Autodesk Inventor part; units mm, degrees
ref_plane "Work Plane1" through (0, 0, -15) normal (0, 0, 1) x (1, 0, 0)
ref_plane "YZ Plane" through (0, 0, 0) normal (1, 0, 0) x (0, 1, 0)
ref_plane "XZ Plane" through (0, 0, 0) normal (0, 1, 0) x (-1, 0, 0)
sketch "Sketch1" plane through (0, 0, 0) normal (0, 0, 1) x (1, 0, 0)
  line L0 (0, 0) -> (25, 0)
  line L1 (25, 0) -> (25, 40)
  line L2 (25, 40) -> (0, 40)
  line L3 (0, 40) -> (0, 0)
  dimension "d1" = 25
  dimension "d2" = 40
  dimension "d3" = 25
extrude "Extrusion1" add sketch "Sketch1" against normal blind 30
sketch "Sketch2" plane through (25, 0, 0) normal (1, 0, 0) x (0, 0, -1)
  line L0 (0, 0) -> (30, 0)
  circle A0 centre (15, 6.56) radius 2.46
extrude "Extrusion2" cut sketch "Sketch2" against normal blind 30
sketch "Sketch3" plane through (0, 0, 0) normal (-1, 0, 0) x (0, 0, 1)
  line L0 (0, 0) -> (-30, 0)
  line L1 (-25.05, 0) -> (-4.95, 0)
  line L2 (-4.95, 0) -> (-4.95, 33.12)
  line L3 (-4.95, 33.12) -> (-25.05, 33.12)
  line L4 (-25.05, 33.12) -> (-25.05, 0)
  dimension "d11" = 20.1
extrude "Extrusion3" cut sketch "Sketch3" against normal blind 20
sketch "Sketch4" plane through (0, 0, 0) normal (0, -1, 0) x (1, 0, 0)
  line L0 (20, -4.95) -> (20, -25.05)
  line L1 (20, -15) -> (25, -15)
  line L2 (25, 0) -> (25, -30)
  line L3 (20, -8.025) -> (25, -8.025)
  line L4 (25, -8.025) -> (25, -21.975)
  line L5 (25, -21.975) -> (20, -21.975)
  line L6 (20, -21.975) -> (20, -8.025)
  line L7 (20, -8.025) -> (25, -21.975) construction
  line L8 (25, -8.025) -> (20, -21.975) construction
  line L9 (25, -12.54) -> (25, -17.46)
  point P0 (0, 0)
  point P1 (22.5, -15)
  dimension "d14" = 13.95
extrude "Extrusion4" add sketch "Sketch4" along normal blind 15
sketch "Sketch5" plane through (20, 0, 0) normal (-1, 0, 0) x (0, 0, 1)
  circle A0 centre (-15, 6.56) radius 2.46
  circle A1 centre (-15, 6.56) radius 4.7025
  circle A2 centre (-15, 6.56) radius 2.46
  circle A3 centre (-15, 6.56) radius 2.46
  point P0 (0, 0)
  dimension "d17" = 9.405
extrude "Extrusion5" cut sketch "Sketch5" against normal blind 2.1
sketch "Sketch6" plane through (25, 0, 0) normal (1, 0, 0) x (0, 0, -1)
  circle A0 centre (15, 6.56) radius 4.7025
  line L0 (15, 6.56) -> (15, 23.56)
  circle A1 centre (15, 23.56) radius 2.46
  point P0 (0, 0)
  dimension "d20" = 17
  dimension "d21" = 4.92
extrude "Extrusion6" cut sketch "Sketch6" against normal blind 10 contours A1
sketch "Sketch7" plane through (20, 0, 0) normal (-1, 0, 0) x (0, 0, 1)
  circle A0 centre (-15, 23.56) radius 2.46
  circle A1 centre (-15, 23.56) radius 4.7025
  point P0 (0, 0)
  dimension "d24" = 9.405
extrude "Extrusion7" cut sketch "Sketch7" against normal blind 2.1
sketch "Sketch9" plane through (25, 0, 0) normal (1, 0, 0) x (0, 0, -1)
  circle A0 centre (15, 6.56) radius 2.46
  circle A1 centre (15, 6.56) radius 2.46
  circle A2 centre (15, 23.56) radius 2.46
  circle A3 centre (15, 23.56) radius 2.46
  line L0 (30, 40) -> (30, 0)
  line L1 (30, 0) -> (30, 40)
  line L2 (30, 40) -> (0, 40)
  line L3 (0, 40) -> (0, 0)
  line L4 (0, 0) -> (8.025, 0)
  line L5 (21.975, 0) -> (21.975, -15)
  line L6 (21.975, -15) -> (8.025, -15)
  line L7 (8.025, -15) -> (8.025, 0)
  line L8 (0, 0) -> (8.025, 0)
  line L9 (21.975, 0) -> (30, 0)
extrude "Extrusion8" add sketch "Sketch9" along normal blind 5
sketch "Sketch10" plane through (0, 40, 0) normal (0, 1, 0) x (1, 0, 0)
  line L0 (0, 30) -> (30, 30)
  line L1 (30, 0) -> (0, 0)
  line L2 (0, 30) -> (30, 30)
  line L3 (30, 30) -> (30, 0)
  line L4 (30, 0) -> (0, 0)
  line L5 (0, 0) -> (0, 30)
extrude "Extrusion9" add sketch "Sketch10" along normal blind 30
sketch "Sketch12" plane through (30, 0, 0) normal (1, 0, 0) x (0, 0, -1)
  circle A0 centre (15, 6.56) radius 2.46
  line L0 (15, 6.56) -> (15, 15.06)
  circle A1 centre (15, 15.06) radius 2.525
  point P0 (0, 0)
  dimension "d31" = 8.5
  dimension "d33" = 5.05
extrude "Extrusion10" cut sketch "Sketch12" against normal blind 30 contours A1
sketch "Sketch14" plane through (0, 0, 0) normal (0, 0, 1) x (1, 0, 0)
  line L0 (30, 70) -> (0, 70)
  line L1 (0, 70) -> (0, 85)
  line L2 (-15, 100) -> (-23, 100)
  line L3 (30, 0) -> (30, 70)
  line L4 (30, 100) -> (30, 70)
  arc A0 (0, 85) -> (-15, 100) centre (-15, 85) ccw
  line L5 (-23, 120) -> (15, 120)
  line L6 (-20.5, 118) -> (-18, 110)
  line L7 (-20.5, 118) -> (-23, 120)
  line L8 (-20.5, 102) -> (-18, 110)
  line L9 (-20.5, 102) -> (-23, 100)
  line L10 (30, 105) -> (15, 120)
  line L11 (30, 105) -> (30, 100)
  point P0 (0, 0)
  point P1 (0, 100)
  dimension "d47" = 30
  dimension "d54" = 15
  dimension "d60" = 20
extrude "Extrusion12" add sketch "Sketch14" against normal blind 30
sketch "Sketch15" plane through (0, 0, -25.05) normal (-1, 0, 0) x (0, 0, 1)
  line L0 (0, 33.12) -> (20.1, 33.12)
  line L1 (20.1, 33.12) -> (20.1, 0)
  line L2 (0, 33.12) -> (20.1, 33.12)
  line L3 (20.1, 33.12) -> (20.1, 31.1)
  line L4 (20.1, 31.1) -> (0, 31.1)
  line L5 (0, 31.1) -> (0, 33.12)
  point P0 (25.05, 0)
  dimension "d57" = 2.02
extrude "Extrusion13" add sketch "Sketch15" against normal blind 20
sketch "Sketch19" plane through (0, 0, 0) normal (0, 0, 1) x (1, 0, 0)
  arc A0 (0, 85) -> (-15, 100) centre (-15, 85) ccw
  arc A1 (0, 85) -> (-15, 100) centre (-15, 85) ccw
  line L0 (-15, 100) -> (-23, 100)
  line L1 (-15, 100) -> (-23, 100)
  line L2 (-23, 100) -> (-20.5, 102)
  line L3 (-23, 100) -> (-20.5, 102)
  line L4 (-20.5, 102) -> (-18, 110)
  line L5 (-20.5, 102) -> (-18, 110)
  line L6 (-18, 110) -> (-20.5, 118)
  line L7 (-18, 110) -> (-20.5, 118)
  line L8 (-23, 120) -> (15, 120)
  line L9 (-20.5, 118) -> (-23, 120)
  line L10 (-23, 120) -> (15, 120)
  line L11 (15, 120) -> (30, 105)
  line L12 (15, 120) -> (30, 105)
  line L13 (30, 105) -> (30, 85)
  line L14 (30, 0) -> (30, 105)
  line L15 (0, 85) -> (30, 85)
  point P0 (0, 0)
extrude "Extrusion14" add sketch "Sketch19" along normal blind 15
ref_plane "Work Plane1" through (0, 0, -15) normal (0, 0, 1) x (1, 0, 0)
mirror "Mirror1" about plane through (0, 0, -15) normal (0, 0, 1) of "Extrusion14"
properties part number "16mm_x_60mm"
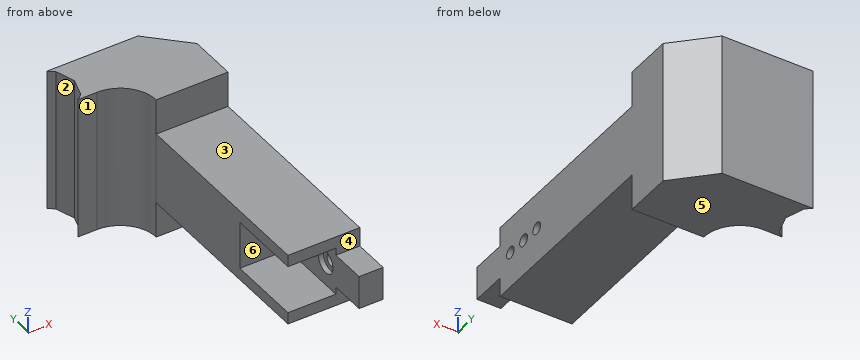
Source: CAD feature listing. Evaluate the final solid. Frame: model axes, mm. Face numbers are marked on the shaded views. A direction names the side the tool comes from. Coordinates: 2 decimals unless noted, no trailing zeros. Order: outer loops, then holes, each group sorted by start corner. A loop starts at its lowest first (then second) coordinate and runs counter-clockwise, first axis right, second up. Notation, with made-up numbers: M -3.75,21.25 L 25.25,21.25 A12 cw 25.25,37.25 Z; hole C 59.25,44.5 d7. An arc over 180 degrees is marked long. Write each question's results on one line, items separated by ' | '. Start each with the question number.
1) Access query for the marked faces 1, 2 and 3. Directions: +Z, -Z, +X, -X, +Y, -Y. A direction counts if a zero-diameter tool reaches every point of the face in a straight line with its end or side. Return the directions, or none.
2) Section query D-D (x = 4). Return the cut outline in (y, z), plus the area to 3 significant figures.
3) Contact query for flat-ended pins moving along their axis: pin 1 Ø10 at (x, y) = (10.5, 13.5) entering from -Z; pin 2 Ø8 at (x, y) = (23, -9) entering from +Z (3 decimals); pin 3 Ø10 at (x, z) = (8, -19.5) entering from -Y. Output: stop coordinate, or through.
4) Section query B-B (z = -15). Give the number of separate pieces and of enclosed holes in the cut face, plus the area to 3 significant figures.
5) Section query A-A (y = 15.06). Return the cut outline in (x, z) (3 decimals).
6) Section query C-C (z = -3). Return the cut outline in (x, y), plus the area to 3 significant figures.
7) Line query: line 1 (Y direction, x = 20.9, z = -15) (1 decimal); line 2 (Y direction, x = 28, z = -15) (3 decimals); line 3 (Z direction, x = 27, y = 15). Output: solid intervals per line, ascending. Write a range as from..to.
8) Draft query along Z for the marked faces 4, 5 and 6. Return one class per face: released by +Z, released by -Z, zero draft, split by the parting line, or undercut.
Answers:
1) face 1: +Z, -Z, -X, -Y | face 2: +Z, -Z, -X | face 3: +Z, +X, -X, -Y
2) outline: M 0,-30 L 85,-30 L 85,-45 L 120,-45 L 120,15 L 85,15 L 85,0 L 0,0 L 0,-4.95 L 31.1,-4.95 L 31.1,-25.05 L 0,-25.05 Z | area: 4,020 mm^2
3) pin 1: stops at z = -30 | pin 2: stops at z = -8.025 | pin 3: stops at y = 31.1
4) separate pieces: 4 | enclosed holes: 0 | area: 3,290 mm^2
5) outline: M 0,-30 L 30,-30 L 30,-17.525 L 20,-17.525 L 20,-25.05 L 0,-25.05 Z; M 0,-4.95 L 20,-4.95 L 20,-12.475 L 30,-12.475 L 30,0 L 0,0 Z
6) outline: M -23,100 L -15,100 A15 cw 0,85 L 0,0 L 30,0 L 30,105 L 15,120 L -23,120 L -20.5,118 L -18,110 L -20.5,102 Z | area: 3,930 mm^2
7) line 1: y = -15..1.9, 11.3..12.5, 17.6..18.9, 28.3..114.1 | line 2: y = -15..4.1, 9.02..12.535, 17.585..21.1, 26.02..107 | line 3: z = -30..-17.52, -12.48..0
8) face 4: zero draft | face 5: released by -Z | face 6: undercut
